Verification items for the finished model (mm, model axes). Coordinates: 2 decimals unless noted, no trailing zeros. Order: outer loops, then holes, each group sorted by start corner. A loop starts at its lowest first (then second) coordinate and runs counter-clockwise, first axis right, second up. Notation, with made-up numbers: (82, 2) - (110, 2) arc R15 ccw to (110, 12) - close; hole circle Ø11 at (77.25, 5.5). An arc over 180 degrees is marked (long way). Answer as CSV lines item,"result". Start each with the question number.
1. Section check B-B (y = 2.25). Count the separate pieces of the cut face and the enclosed holes in it, and give its area (3 significant figures).
2. Go/stop test with flat-tipped pins: pin 1 (1 mm diameter, centred on x = -32, y = 1.5, fed in from +Z); pin 2 (2 mm diameter, centred on x = -53, z = -19, fed in from +Y); pin 3 (0.9 mm diameter, centred on x = -51.5, y = 1.5, fed in from +Z); pin 4 (2 mm diameter, centred on x = -46, y = 0.5, fed in from -Z). Record where each tip stops, or that it passes through.
3. Section check A-A (x = -9). Record the cut outline in (y, z), and give its area (3 significant figures).
4. Material ranges on L1, parallel to X at y = 1.3, z = 5; L2, parallel to Z at x = -63, y = 3.3; L3, parallel to X at y = 1.8, z = -11, recorded low to high. Write a range as [from, to].
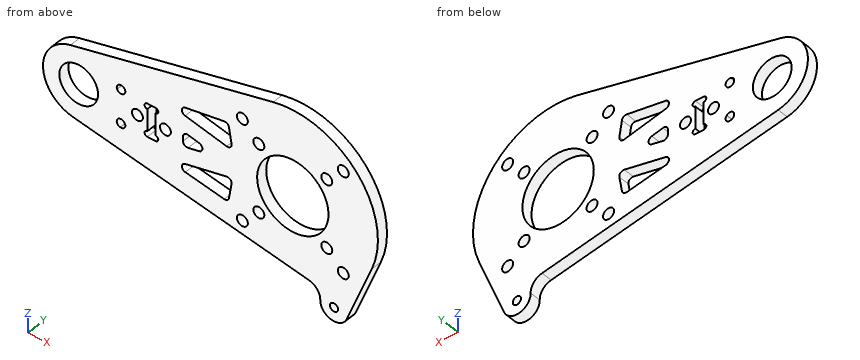
from build123d import *

# Parameters (mm, degrees)
SKETCH_1_R          = 7.05
SKETCH_1_R_2        = 1.5
SKETCH_1_R_3        = 2
SKETCH_1_R_4        = 13
EXTRUDE_1_DEPTH     = 4
SKETCH_4_R          = 2
SKETCH_4_W          = 3
SKETCH_4_H          = 12
CUT_EXTRUDE_7_DEPTH = 99.505076011
SKETCH_8_R          = 1
CUT_EXTRUDE_6_DEPTH = 99.505076011
CUT_EXTRUDE_8_DEPTH = 99.505076011
FILLET_1_R          = 1.5


with BuildPart() as part:
    # 草图1 → 凸台-拉伸1 (new body)
    with BuildSketch(Plane(origin=(0, 0, 0), x_dir=(1, 0, 0), z_dir=(0, 1, 0))):
        with BuildLine():
            Line((-80.166666667, 12.818172863), (5.835638785, 27.355215737))
            ThreePointArc((5.835638785, 27.355215737), (8.855550352, 29.098982843), (10.001152726, 32.392641112))
            ThreePointArc((10.001152726, 32.392641112), (14.001538866, 37.399293353), (19.642183216, 34.3574539))
            Line((19.642183216, 34.3574539), (28.781535937, 11.516214183))
            ThreePointArc((28.781535937, 11.516214183), (23.478372246, -20.242678595), (-7.153846154, -30.163263835))
            Line((-7.153846154, -30.163263835), (-81, -12.649110641))
            ThreePointArc((-81, -12.649110641), (-90.993045962, 0.425154819), (-80.166666667, 12.818172863))
        make_face()
        with Locations(Location((-78, 0, 0), (0, 0, 270))):
            Circle(SKETCH_1_R, mode=Mode.SUBTRACT)
        with Locations(Location((15, 32.5, 0), (0, 0, 270))):
            Circle(SKETCH_1_R_2, mode=Mode.SUBTRACT)
        with Locations(Location((-18.384776311, 18.384776311, 0), (0, 0, 270))):
            Circle(SKETCH_1_R_3, mode=Mode.SUBTRACT)
        with Locations(Location((18.384776311, 18.384776311, 0), (0, 0, 270))):
            Circle(SKETCH_1_R_3, mode=Mode.SUBTRACT)
        with Locations(Location((18.384776311, -18.384776311, 0), (0, 0, 270))):
            Circle(SKETCH_1_R_3, mode=Mode.SUBTRACT)
        with Locations(Location((-18.384776311, -18.384776311, 0), (0, 0, 270))):
            Circle(SKETCH_1_R_3, mode=Mode.SUBTRACT)
        with Locations(Location((-12.374368671, 12.374368671, 0), (0, 0, 270))):
            Circle(SKETCH_1_R_3, mode=Mode.SUBTRACT)
        with Locations(Location((12.374368671, 12.374368671, 0), (0, 0, 270))):
            Circle(SKETCH_1_R_3, mode=Mode.SUBTRACT)
        with Locations(Location((12.374368671, -12.374368671, 0), (0, 0, 270))):
            Circle(SKETCH_1_R_3, mode=Mode.SUBTRACT)
        with Locations(Location((-12.374368671, -12.374368671, 0), (0, 0, 270))):
            Circle(SKETCH_1_R_3, mode=Mode.SUBTRACT)
        with Locations(Location((0, 0, 0), (0, 0, 270))):
            Circle(SKETCH_1_R_4, mode=Mode.SUBTRACT)
    extrude(amount=EXTRUDE_1_DEPTH)

    # 草图4 → 切除-拉伸7 (cut, through all)
    with BuildSketch(Plane(origin=(0, 4, 0), x_dir=(1, 0, 0), z_dir=(0, 1, 0))):
        with Locations(Location((-56.6, 0, 0), (0, 0, 270))):
            Circle(SKETCH_4_R)
        with Locations(Location((-46.4, 0, 0), (0, 0, 270))):
            Circle(SKETCH_4_R)
        with Locations((-51.5, 0)):
            Rectangle(SKETCH_4_W, SKETCH_4_H)
    extrude(amount=-CUT_EXTRUDE_7_DEPTH, mode=Mode.SUBTRACT)

    # 草图8 → 切除-拉伸6 (cut, through all)
    with BuildSketch(Plane(origin=(0, 4, 0), x_dir=(1, 0, 0), z_dir=(0, 1, 0))):
        with Locations((-53, 5)):
            Circle(SKETCH_8_R)
        with Locations((-53, -5)):
            Circle(SKETCH_8_R)
        with Locations((-50, -5)):
            Circle(SKETCH_8_R)
        with Locations((-50, 5)):
            Circle(SKETCH_8_R)
    extrude(amount=-CUT_EXTRUDE_6_DEPTH, mode=Mode.SUBTRACT)

    # 草图9 → 切除-拉伸8 (cut, through all)
    with BuildSketch(Plane(origin=(0, 4, 0), x_dir=(1, 0, 0), z_dir=(0, 1, 0))):
        Polygon((-23.506360694, 14.282031751), (-21.937410968, 5), (-46.887877974, 10.329833989), align=None)
        Polygon((-46.887877974, -10.329833989), (-23.506360694, -14.282031751), (-21.937410968, -5), align=None)
        with BuildLine():
            Line((-64.836719159, 7.29592609), (-58.661742218, 8.339687697))
            Line((-58.661742218, 8.339687697), (-63.252034039, 3))
            ThreePointArc((-63.252034039, 3), (-63.880043564, 5.208582364), (-64.836719159, 7.29592609))
        make_face()
        with BuildLine():
            Line((-58.661742218, -8.339687697), (-63.252034039, -3))
            ThreePointArc((-63.252034039, -3), (-63.880043564, -5.208582364), (-64.836719159, -7.29592609))
            Line((-64.836719159, -7.29592609), (-58.661742218, -8.339687697))
        make_face()
        Polygon((-40, 2.723099806), (-27.252396227, 0), (-40, -2.723099806), align=None)
    extrude(amount=-CUT_EXTRUDE_8_DEPTH, mode=Mode.SUBTRACT)

    # 圆角1
    fillet_1_edges = [part.edges().sort_by_distance(p)[0] for p in [
        (-46.887877974, 2, 10.329833989),
        (-21.937410968, 2, 5),
        (-23.506360694, 2, 14.282031751),
        (-63.252034039, 2, -3),
        (-64.836719159, 2, -7.29592609),
        (-58.661742218, 2, -8.339687697),
        (-40, 2, 2.723099806),
        (-40, 2, -2.723099806),
        (-27.252396227, 2, 0),
        (-64.836719159, 2, 7.29592609),
        (-63.252034039, 2, 3),
        (-58.661742218, 2, 8.339687697),
        (-46.887877974, 2, -10.329833989),
        (-23.506360694, 2, -14.282031751),
        (-21.937410968, 2, -5),
    ]]
    fillet(fillet_1_edges, radius=FILLET_1_R)


solid = part.part
Evaluation:
1,separate pieces,"1"
1,enclosed holes,"19"
1,area,"4,070 mm²"
2,pin 1,"stops at z = 24.39"
2,pin 2,"passes through"
2,pin 3,"stops at z = 19.75"
2,pin 4,"stops at z = -18.76"
3,outline,"(0, -24.85) - (4, -24.85) - (4, -9.38) - (0, -9.38) - close; (0, 9.38) - (4, 9.38) - (4, 29.73) - (0, 29.73) - close"
3,area,"143 mm²"
4,L1,"x = [-90, -82.97], [-73.03, -63.66], [-61.54, -54], [-49, -12], [12, 30.59]"
4,L2,"z = [-15.72, -7.6], [-4.61, 4.61], [7.6, 16.92]"
4,L3,"x = [-84.93, -40.15], [-22.95, -13.83], [-10.92, -6.93], [6.93, 10.92], [13.83, 28.98]"
